from build123d import *

# Parameters (mm, degrees)
SKETCH1_R           = 1
BOSS_EXTRUDE1_DEPTH = 5
FILLET1_R           = 0.75


with BuildPart() as part:
    # Sketch1 → Boss-Extrude1 (new body)
    with BuildSketch(Plane(origin=(0, 0, 0), x_dir=(1, 0, 0), z_dir=(0, 1, 0))):
        with BuildLine():
            Line((17.35965567, 10.202030332), (29.447075717, 10.202030332))
            ThreePointArc((29.447075717, 10.202030332), (31.66677099, 11.984583247), (34.447841937, 11.376153807))
            ThreePointArc((34.447841937, 11.376153807), (35.368803472, 10.219084334), (35.659625363, 8.769117942))
            Line((35.659625363, 8.769117942), (35.368803472, 6.25123518))
            ThreePointArc((35.368803472, 6.25123518), (35.604797827, 4.927222302), (36.70788952, 4.157877025))
            Line((36.70788952, 4.157877025), (48.178757035, 2.245683648))
            Line((48.178757035, 2.245683648), (47.58886704, -1.292949037))
            ThreePointArc((47.58886704, -1.292949037), (47.751350099, -2.119984122), (48.327597047, -2.73506723))
            Line((48.327597047, -2.73506723), (53.807205044, -7.165448567))
            Line((53.807205044, -7.165448567), (62.256251854, -10.114363821))
            ThreePointArc((62.256251854, -10.114363821), (63.012595107, -10.242357854), (63.768803253, -10.11356799))
            Line((63.768803253, -10.11356799), (64.838933553, -6.777694818))
            ThreePointArc((64.838933553, -6.777694818), (64.82438131, -6.262093226), (64.449505937, -5.907797834))
            Line((64.449505937, -5.907797834), (55.769751742, -2.596216357))
            Line((55.769751742, -2.596216357), (46.89988124, 9.654677352))
            Line((46.89988124, 9.654677352), (36.858577183, 11.505687421))
            Line((36.858577183, 11.505687421), (34.863073504, 15.401227244))
            Line((34.863073504, 15.401227244), (19.873257266, 15.461670051))
            Line((19.873257266, 15.461670051), (10.836196027, 6.49719565))
            Line((10.836196027, 6.49719565), (-0.977680405, 4.492963372))
            Line((-0.977680405, 4.492963372), (0, 0))
            Line((0, 0), (17.101259036, 2.779786934))
            Line((17.101259036, 2.779786934), (17.35965567, 10.202030332))
        make_face()
        with Locations((59.08099239, -6.537460134)):
            Circle(SKETCH1_R, mode=Mode.SUBTRACT)
        with Locations((23.534477486, 11.983797813)):
            Circle(SKETCH1_R, mode=Mode.SUBTRACT)
        with Locations((4.870081777, 2.779786934)):
            Circle(SKETCH1_R, mode=Mode.SUBTRACT)
        with Locations((42.49591928, 5.349768569)):
            Circle(SKETCH1_R, mode=Mode.SUBTRACT)
    extrude(amount=BOSS_EXTRUDE1_DEPTH)

    # Fillet1
    fillet1_edges = [part.edges().sort_by_distance(p)[0] for p in [
        (17.101259036, 2.5, -2.779786934),
        (0, 2.5, 0),
        (-0.977680405, 2.5, -4.492963372),
        (19.873257266, 2.5, -15.461670051),
        (34.863073504, 2.5, -15.401227244),
    ]]
    fillet(fillet1_edges, radius=FILLET1_R)


solid = part.part
Check sheet for the modelled part. Datum: model origin and axes. Units: mm. A direction names the side the tool comes from. Round coordinates to 2 decimals unless told otherwise and drop trailing zeros. Order: outer loops, then holes, each group sorted by start corner. A loop starts at its lowest first (then second) coordinate and runs counter-clockwise, first axis right, second up.
(1) Cross-section at B-B, the plane y = 1.05. State how many separate pieces and enclosed holes the cut face has, and give its area (3 significant figures).
(2) Cross-section at A-A, the plane z = -7.5. Enter the section's corners in (x, y), and give its area (3 significant figures).
(3) Cross-section at D-D, the plane x = 7. Enter the section's corners in (y, z).
(4) Access from +Z, -Z, +X, -X, +Y, -Y to the whole of each face (thin tool, end or side, straight path). Record for faces 5 (the flat face through (23, 2, -10.202)), 6 (the flat face through (35.516, 2.465, -7.528)), 7 (the flat face through (60.17, 2.465, 4.275)).
(5) Draft check along X on faces 1 (the flat face through (64.296, 2.465, 8.469)), 2 (the flat face through (47.888, 2.465, -0.501)), 3 (the flat face through (37, 0, -6)), 4 (the flat face through (-0.486, 2.465, -2.231)). Enter one of: pulls with the +X half, pulls with the -X half, needs draft (parallel to the pull), parting line crosses it, or undercut.
(6) Scan lines: probe 1 along X at (y, z) = (3.1, -11.75); probe 2 along Z at (x, y) = (22, 1.6); probe 3 along X at (y, z) = (3.7, -8). Record each from-to range of solid material in increasing order.
(7) Cross-section at C-C, the plane x = 40.5. Enter the section's corners in (y, z), and give its area (3 significant figures).
(8) Go/stop test with flat-tipped pins: P1, Ø3, axis at x = 6.5, y = 4.5, coming from the -Z side; P2, Ø3, axis at x = 25, y = 2.5, coming from the +Z side. Record where each tip stops, or that it passes through.
Check sheet entries:
1. separate pieces: 1
1. enclosed holes: 4
1. area: 371 mm2
2. outline: (11.85, 0) - (17.27, 0) - (17.27, 5) - (11.85, 5) - close; (35.51, 0) - (48.46, 0) - (48.46, 5) - (35.51, 5) - close
2. area: 91.8 mm2
3. outline: (0, -5.85) - (5, -5.85) - (5, -1.14) - (0, -1.14) - close
4. face 5: +Z, +Y, -Y
4. face 6: +Y, -Y
4. face 7: -Z, +X, +Y, -Y
5. face 1: pulls with the +X half
5. face 2: undercut
5. face 3: needs draft
5. face 4: pulls with the -X half
6. probe 1: x = 16.13 to 22.56, 24.51 to 31, 33.84 to 36.73
6. probe 2: z = -15.45 to -10.2
6. probe 3: x = 12.35 to 17.28, 35.57 to 48.1
7. outline: (0, -10.83) - (5, -10.83) - (5, -3.53) - (0, -3.53) - close
7. area: 36.5 mm2
8. P1: stops at z = -6.02
8. P2: stops at z = -10.2
